Source: CAD feature listing. Evaluate the final solid. Frame: model axes, mm. A direction names the side the tool comes from. Give positions to 0.01 mm unless a question says otherwise; leave off trailing zeros. Loops run counter-clockwise (first coordinate to the right, second up) from the corner with the lowest first, then second, coordinate; pieces in that order, holes last. Notation, with made-up numbers: (62, 22) -> (69, 22) arc R26 cw to (69, 61) -> close; hole circle Ø11 at (0, 0). An arc over 180 degrees is marked (long way). Put each result on its own line as item: value.
```python
from build123d import *

# Parameters (mm, degrees)
SZKIC13_R                   = 1.55
DODANIE_WYCI_GNI_CIE3_DEPTH = 6
SZKIC15_R                   = 2.6
WYTNIJ_WYCI_GNI_CIE3_DEPTH  = 226.954786153
SZKIC17_R                   = 1.550000001
WYTNIJ_WYCI_GNI_CIE4_DEPTH  = 10
WYTNIJ_WYCI_GNI_CIE5_START  = -10
WYTNIJ_WYCI_GNI_CIE5_DEPTH  = 10
SZKIC19_R                   = 1.55
WYTNIJ_WYCI_GNI_CIE6_DEPTH  = 10


with BuildPart() as part:
    # Szkic13 → Dodanie-wyciągnięcie3 (new body)
    with BuildSketch(Plane(origin=(79.289240162, 6, 79.289240162), x_dir=(-1, 0, 0), z_dir=(0, 1, 0))):
        with BuildLine():
            Line((-25.202360127, 55.749482984), (-3.551339243, 75.782812897))
            ThreePointArc((-3.551339243, 75.782812897), (10.580158874, 75.234396129), (10.031742107, 61.102898012))
            Line((10.031742107, 61.102898012), (-7.738470336, 44.660415673))
            ThreePointArc((-7.738470336, 44.660415673), (-10.310546151, 37.859798404), (-7.5965153, 31.114577446))
            Line((-7.5965153, 31.114577446), (14.933655573, 7.152316182))
            ThreePointArc((14.933655573, 7.152316182), (13.398314201, -14.533932284), (-8.183163771, -11.908964821))
            Line((-8.183163771, -11.908964821), (-15.992976767, -1.557886957))
            ThreePointArc((-15.992976767, -1.557886957), (-22.556998647, 4.097640789), (-30.974241603, 6.152244974))
            ThreePointArc((-30.974241603, 6.152244974), (-39.464828567, 4.425597836), (-46.243228353, -0.971130216))
            Line((-46.243228353, -0.971130216), (-54.448570559, -11.011566026))
            ThreePointArc((-54.448570559, -11.011566026), (-76.115608669, -12.797652588), (-76.808825852, 8.931822684))
            Line((-76.808825852, 8.931822684), (-53.366371193, 32.002364161))
            ThreePointArc((-53.366371193, 32.002364161), (-50.392809402, 38.637264273), (-52.699229936, 45.532508544))
            Line((-52.699229936, 45.532508544), (-69.818454156, 62.651732764))
            ThreePointArc((-69.818454156, 62.651732764), (-69.818454156, 76.793868387), (-55.676318532, 76.793868387))
            Line((-55.676318532, 76.793868387), (-34.818454156, 55.936004011))
            ThreePointArc((-34.818454156, 55.936004011), (-30.049036911, 53.851185216), (-25.202360127, 55.749482984))
        make_face()
        with Locations((-62.747386344, 69.722800575)):
            Circle(SZKIC13_R, mode=Mode.SUBTRACT)
        with Locations(Location((3.855577347, -2.960852601, 0), (0, 0, 180))):
            Circle(SZKIC13_R, mode=Mode.SUBTRACT)
        with Locations(Location((3.240201432, 68.442855454, 0), (0, 0, 180))):
            Circle(SZKIC13_R, mode=Mode.SUBTRACT)
        with Locations((-66.131258172, -1.603335049)):
            Circle(SZKIC13_R, mode=Mode.SUBTRACT)
    extrude(amount=-DODANIE_WYCI_GNI_CIE3_DEPTH)

    # Szkic15 → Wytnij-wyciągnięcie3 (cut, through all)
    with BuildSketch(Plane(origin=(0, 0, 0), x_dir=(0.707106781186548, 0, 0.7071067811865471), z_dir=(0, -1, 0))):
        with Locations(Location((145.72647023, 5.947865628, 0), (0, 0, 315))):
            Circle(SZKIC15_R)
        with Locations(Location((150.579295842, 10.992673214, 0), (0, 0, 315))):
            Circle(SZKIC15_R)
        with Locations(Location((161.581579785, -9.30387201, 0), (0, 0, 315))):
            Circle(SZKIC15_R)
        with Locations(Location((166.434405397, -4.259064425, 0), (0, 0, 315))):
            Circle(SZKIC15_R)
    extrude(amount=-WYTNIJ_WYCI_GNI_CIE3_DEPTH, mode=Mode.SUBTRACT)

    # Szkic17 → Wytnij-wyciągnięcie4 (cut)
    with BuildSketch(Plane(origin=(0, 0, 0), x_dir=(0.7071067811865479, 0, 0.7071067811865472), z_dir=(0, -1, 0))):
        with Locations(Location((109.947888172, 10.585151125, 0), (0, 0, 225))):
            Circle(SZKIC17_R)
        with Locations(Location((167.602832009, -44.875713015, 0), (0, 0, 225))):
            Circle(SZKIC17_R)
    extrude(amount=-WYTNIJ_WYCI_GNI_CIE4_DEPTH, mode=Mode.SUBTRACT)

    # Szkic18 → Wytnij-wyciągnięcie5 (cut)
    with BuildSketch(Plane.XZ.offset(WYTNIJ_WYCI_GNI_CIE5_START)):
        with BuildLine():
            Line((116.622706822, 84.5530515), (115.830023537, 116.303650978))
            Line((115.830023537, 116.303650978), (102.834025094, 115.981122728))
            Line((102.834025094, 115.981122728), (103.61834975, 84.184343244))
            ThreePointArc((103.61834975, 84.184343244), (106.883098894, 85.118528612), (110.263481765, 85.441485136))
            ThreePointArc((110.263481765, 85.441485136), (113.481855081, 85.274710056), (116.622706822, 84.5530515))
        make_face()
    extrude(amount=WYTNIJ_WYCI_GNI_CIE5_DEPTH, mode=Mode.SUBTRACT)

    # Szkic19 → Wytnij-wyciągnięcie6 (cut)
    with BuildSketch(Plane.XZ):
        with Locations((104.20638679, 125.017952482)):
            Circle(SZKIC19_R)
        with Locations((114.20638679, 125.017952482)):
            Circle(SZKIC19_R)
    extrude(amount=-WYTNIJ_WYCI_GNI_CIE6_DEPTH, mode=Mode.SUBTRACT)


solid = part.part
```
(1) First-contact query: P1, Ø4, axis at x = 120.83, z = 107.68, coming from the +Y side; P2, Ø8.5, axis at x = 98.84, z = 107.25, coming from the +Y side. Flat tips, straight axial feed; report the tip coordinate or a pass-through.
Calculated:
P1: passes through
P2: stops at y = 6
(2) Draft query along Z for faces 4 (the cylindrical face through (121.48, 3.04, 82.15)), 5 (the flat face through (144.541, 3.042, 99.595)), 6 (the flat face through (121, 6, 100)). Return one class per face: released by +Z, released by -Z, zero draft, split by the parting line, or undercut.
Calculated:
face 4: released by -Z
face 5: undercut
face 6: zero draft
(3) Section A-A on x = 84. Return loops of the section in (y, z).
Calculated:
outline: (0, 64.02) -> (6, 64.02) -> (6, 107.33) -> (0, 107.33) -> close; (0, 126.75) -> (6, 126.75) -> (6, 154) -> (0, 154) -> close
(4) Reachability of faces 1 (the cylindrical face through (142.37, 3.04, 147.5)), 2 (the flat face through (140.428, 3.042, 133.262)), 3 (the flat face through (75.78, 3.04, 98.59)) from +Z, -Z, +X, -X, +Y, -Y: full face, straight path, thin tool, end or side. Return the list, or none.
Calculated:
face 1: +Y, -Y
face 2: +X, +Y, -Y
face 3: -X, +Y, -Y
(5) Section B-B on y = 3.55. Give the number of separate pieces and of enclosed holes in the cut face, then the cut area to 3 significant figures.
Calculated:
separate pieces: 1
enclosed holes: 12
area: 4,850 mm²
(6) Section C-C on z = 100. Return loops of the section in (x, y), then the cut area to 3 significant figures.
Calculated:
outline: (77.1, 0) -> (103.23, 0) -> (103.23, 6) -> (77.1, 6) -> close; (116.24, 0) -> (144.13, 0) -> (144.13, 6) -> (116.24, 6) -> close
area: 324 mm²
(7) Line query: probe 1 along X at (y, z) = (0.5, 114); probe 2 along X at (y, z) = (3.7, 85); probe 3 along X at (y, z) = (5.45, 149.5). Output: solid intervals per line, ascending. Write a range as from..to.
Calculated:
probe 1: x = 89.06..96.11, 101.29..102.88, 115.89..118.19, 123.21..130.7
probe 2: x = 63.19..68.73, 71.79..103.6, 116.61..158.52
probe 3: x = 66.21..88.86, 128.38..140.57, 143.51..152.02
(8) Section D-D on z = 122. Return loops of the section in (x, y).
Calculated:
outline: (88.4, 0) -> (130.33, 0) -> (130.33, 6) -> (88.4, 6) -> close
